Geometry check sheet. Reference: the model listing, model coordinates, mm. A direction names the side the tool comes from. Give positions to 0.01 mm unless a question says otherwise; leave off trailing zeros. Loops run counter-clockwise (first coordinate to the right, second up) from the corner with the lowest first, then second, coordinate; pieces in that order, holes last.
1. Cross-section at B-B, the plane y = 18. Record the cut outline in (x, z).
2. Release check for a two-part mould opening along X. For faces 1 (the cylindrical face through (10, 18, 3)), 2 (the flat face through (61.7, 19, 3)), 3 (the flat face through (13, 0, 3)) record: +X half, -X half, draft (parallel to the pull), parting line (faces both ways), or undercut.
3. Tool access check on faces 4 (the flat face through (0, 15, 3)), 5 (the flat face through (5, 3, 3)). Record the directions out of +Z, -Z, +X, -X, +Y, -Y that give a thin tool (end or side, any length) a straight path to the whole face; none if there is none.
4. Go/stop test with flat-tipped pins: pin 1 Ø1.5 at (x, z) = (48, 3) entering from -Y; pin 2 Ø3 at (y, z) = (3, 4) entering from +X. Record where each tip stops, or that it passes through.
5. Cross-section at A-A, the plane x = 43.7. Record the cut outline in (y, z), plus the area to 3 significant figures.
6. Material ranges on L1, parallel to X at y = 1, z = 5.4; L2, parallel to Y at x = 43.7, z = 2.65; L3, parallel to X at y = 14, z = 1.95, recorded low to high.
7. Cross-section at D-D, the plane x = 18. Record the cut outline in (y, z), plus the area to 3 significant figures.
8. Cross-section at C-C, the plane z = 1.15. Record the cut outline in (x, y), plus the area to 3 significant figures.
from build123d import *

# Parameters (mm, degrees)
ESQUISSE1_R        = 8
BOSS_EXTRU_1_DEPTH = 6


with BuildPart() as part:
    # Esquisse1 → Boss.-Extru.1 (new body)
    with BuildSketch(Plane.XY):
        Polygon((0, 0), (0, 31), (61.7, 31), (61.7, 6), (55, 6), (55, 0), (50, 0), (50, 6), (45, 6), (45, 0), (40, 0), (40, 6), (35, 6), (35, 0), (30, 0), (30, 6), (25, 6), (25, 0), (20, 0), (20, 6), (15, 6), (15, 0), (10, 0), (10, 6), (5, 6), (5, 0), align=None)
        with Locations((18, 18)):
            Circle(ESQUISSE1_R, mode=Mode.SUBTRACT)
        with Locations((43.7, 18)):
            Circle(ESQUISSE1_R, mode=Mode.SUBTRACT)
    extrude(amount=BOSS_EXTRU_1_DEPTH)


solid = part.part
Result:
1. outline: (0, 0) - (10, 0) - (10, 6) - (0, 6) - close; (26, 0) - (35.7, 0) - (35.7, 6) - (26, 6) - close; (51.7, 0) - (61.7, 0) - (61.7, 6) - (51.7, 6) - close
2. face 1: undercut
2. face 2: +X half
2. face 3: draft
3. face 4: +Z, -Z, -X, +Y, -Y
3. face 5: +Z, -Z, -Y
4. pin 1: stops at y = 6
4. pin 2: stops at x = 55
5. outline: (0, 0) - (10, 0) - (10, 6) - (0, 6) - close; (26, 0) - (31, 0) - (31, 6) - (26, 6) - close
5. area: 90.0 mm2
6. L1: x = 0 to 5, 10 to 15, 20 to 25, 30 to 35, 40 to 45, 50 to 55
6. L2: y = 0 to 10, 26 to 31
6. L3: x = 0 to 11.07, 24.93 to 36.77, 50.63 to 61.7
7. outline: (6, 0) - (10, 0) - (10, 6) - (6, 6) - close; (26, 0) - (31, 0) - (31, 6) - (26, 6) - close
7. area: 54.0 mm2
8. outline: (0, 0) - (5, 0) - (5, 6) - (10, 6) - (10, 0) - (15, 0) - (15, 6) - (20, 6) - (20, 0) - (25, 0) - (25, 6) - (30, 6) - (30, 0) - (35, 0) - (35, 6) - (40, 6) - (40, 0) - (45, 0) - (45, 6) - (50, 6) - (50, 0) - (55, 0) - (55, 6) - (61.7, 6) - (61.7, 31) - (0, 31) - close; hole circle Ø16 at (18, 18); hole circle Ø16 at (43.7, 18)
8. area: 1,320 mm2
